Could you check a few things on this model? Use its own coordinates, in mm. Give positions to 0.01 mm unless a question says otherwise; leave off trailing zeros. Loops run counter-clockwise (first coordinate to the right, second up) from the corner with the lowest first, then second, coordinate; pieces in that order, holes last. Notation, with made-up numbers: M -5.75,45.25 L 1.25,45.25 A11 ccw 1.25,60.25 Z; hole C -36.5,72.25 d6. An arc over 180 degrees is marked long. Use CSV: the item, a comma, the result in double quotes.
Autodesk Inventor part; units mm, degrees
ref_plane "YZ Plane" through (0, 0, 0) normal (1, 0, 0) x (0, 1, 0)
ref_plane "XZ Plane" through (0, 0, 0) normal (0, 1, 0) x (-1, 0, 0)
ref_plane "XY Plane" through (0, 0, 0) normal (0, 0, 1) x (1, 0, 0)
sketch "Sketch1" plane through (0, 0, 0) normal (0, 1, 0) x (-1, 0, 0)
  line L0 (-12.7, -19.05) -> (12.7, -19.05)
  line L1 (12.7, -19.05) -> (12.7, 19.05)
  line L2 (12.7, 19.05) -> (-12.7, 19.05)
  line L3 (-12.7, 19.05) -> (-12.7, -19.05)
  line L4 (-12.7, -19.05) -> (12.7, 19.05) construction
  line L5 (12.7, -19.05) -> (-12.7, 19.05) construction
  line L6 (12.7, 19.05) -> (0, 19.05)
  line L7 (0, 19.05) -> (0, -19.05)
  line L8 (0, -19.05) -> (12.7, -19.05)
  line L9 (12.7, -19.05) -> (12.7, 19.05)
  line L10 (0, 19.05) -> (-12.7, 6.35)
  line L11 (0, 19.05) -> (17.9605, 19.05) construction
  line L12 (0, -19.05) -> (-12.7, -6.35)
  line L13 (0, -19.05) -> (17.9605, -19.05) construction
  circle A0 centre (6.35, 0) radius 2.1828
  circle A1 centre (-6.35, 0) radius 2.1828
  circle A2 centre (6.35, 12.7) radius 2.1828
  circle A3 centre (6.35, -12.7) radius 2.1828
  point P0 (0, 0)
  point P1 (0, 0)
  point P2 (8.9803, -19.05)
  dimension "d0" = 25.4
  dimension "d1" = 38.1
  dimension "d2" = 135
  dimension "d3" = 135
  dimension "d4" = 4.3656
  dimension "d5" = 4.3656
  dimension "d6" = 4.3656
  dimension "d7" = 4.3656
  dimension "d10" = 12.7
  dimension "d11" = 6.35
  dimension "d12" = 19.05
  dimension "d13" = 19.05
extrude "Extrusion1" add sketch "Sketch1" along normal blind 1.5875 contours L7 L2 L1 L0 | L12 L3 L10 L7
sketch "Sketch2" plane through (0, 1.5875, 0) normal (0, 1, 0) x (1, 0, 0)
  line L0 (12.7, -6.35) -> (12.7, 6.35)
  line L1 (12.7, -6.35) -> (-18.9593, -6.35)
  line L2 (-18.9593, -6.35) -> (-18.9593, -20.186)
  line L3 (-18.9593, -20.186) -> (12.7, -20.186)
  line L4 (12.7, -20.186) -> (12.7, -6.35)
  point P0 (0, 0)
extrude "Extrusion2" cut sketch "Sketch2" against normal blind 25.4
fillet "Fillet1" radius 3.175 5 edges at (12.7, 0.7937, 6.35) (-12.7, 0.7937, 6.35) (12.7, 0.7937, -6.35) (0, 0.7937, -19.05) (-12.7, 0.7937, -19.05)
properties part number "bracket1"
1. I want a section at A-A, the plane z = 0. List the corners of the cut face in (x, y) for me.
Outcome:
outline,"M -12.7,0 L -8.53,0 L -8.53,1.59 L -12.7,1.59 Z; M -4.17,0 L 4.17,0 L 4.17,1.59 L -4.17,1.59 Z; M 8.53,0 L 12.7,0 L 12.7,1.59 L 8.53,1.59 Z"
2. I'm going to push a flat-ended pin straight in: pin 1 Ø3.5 at (x, z) = (-6.35, -12.7) entering from +Y. Where does the tip first touch, or does it pass through?
Outcome:
pin 1,"through"
3. Please list where these lines run through material, in increasing order: line 1 (Z direction, x = -6.35, y = 0.45); line 2 (Z direction, x = -7, y = 1.5); line 3 (X direction, y = 0.3, z = -1).
Outcome:
line 1,"-19.05 to -14.88, -10.52 to -2.18, 2.18 to 6.35"
line 2,"-19.05 to -14.78, -10.62 to -2.08, 2.08 to 6.35"
line 3,"-12.7 to -8.29, -4.41 to 4.41, 8.29 to 12.7"
4. I want a section at D-D, the plane z = -12.7. List the corners of the cut face in (x, y) for me, then the cut area to 3 significant figures.
Outcome:
outline,"M -12.7,0 L -8.53,0 L -8.53,1.59 L -12.7,1.59 Z; M -4.17,0 L 6.35,0 L 6.35,1.59 L -4.17,1.59 Z"
area,"23.3 mm2"
5. If we mould it in two halves opening along X, with no side actions, what happens to faces 1 (the face through (0, 1, 6.35)), 2 (the face through (-4.17, 0.78, -0.1)), 3 (the face through (-12.7, 1, -6))? For each: +X half, -X half, draft (parallel to the pull), parting line (faces both ways), or undercut.
Outcome:
face 1,"draft"
face 2,"undercut"
face 3,"-X half"
6. I want a section at B-B, the plane y = 1.15. List the corners of the cut face in (x, z) for me (3 decimals), then the cut area to 3 significant figures.
Outcome:
outline,"M -12.7,-15.875 A3.175 ccw -9.525,-19.05 L -1.315,-19.05 A3.175 ccw 0.93,-18.12 L 11.77,-7.28 A3.175 ccw 12.7,-5.035 L 12.7,3.175 A3.175 ccw 9.525,6.35 L -9.525,6.35 A3.175 ccw -12.7,3.175 Z; hole C -6.35,-12.7 d4.366; hole C -6.35,0 d4.366; hole C 6.35,0 d4.366"
area,"513 mm2"
7. I want a section at C-C, the plane x = -6.35. List the corners of the cut face in (y, z) for me.
Outcome:
outline,"M 0,-19.05 L 1.59,-19.05 L 1.59,-14.88 L 0,-14.88 Z; M 0,-10.52 L 1.59,-10.52 L 1.59,-2.18 L 0,-2.18 Z; M 0,2.18 L 1.59,2.18 L 1.59,6.35 L 0,6.35 Z"
